Read the model definition and answer for the solid it produces. Units are mm, in the model's axes. A direction names the side the tool comes from. Give positions to 0.01 mm unless a question says otherwise; leave off trailing zeros. Order: outer loops, then holes, each group sorted by start corner. A loop starts at its lowest first (then second) coordinate and runs counter-clockwise, first axis right, second up. Notation, with made-up numbers: (70.25, -19) -> (109.25, -19) arc R23 ccw to (109.25, 3) -> close; hole circle Ø3 at (-25, 69). An arc over 180 degrees is marked (long way). Use one line per item in the form item = value.
```python
from build123d import *

# Parameters (mm, degrees)
SKETCH_1_W               = 44
SKETCH_1_H               = 6.22
EXTRUDE_1_DEPTH          = 0.25
SKETCH_2_W               = 0.25
SKETCH_2_H               = 6.22
EXTRUDE_2_DEPTH          = 1.75
SKETCH_4_W               = 34
SKETCH_4_H               = 0.25
SKETCH_4_W_2             = 9.35
EXTRUDE_3_DEPTH          = 2.25
SKETCH_5_W               = 22.25
SKETCH_5_H               = 2.25
SKETCH_5_W_2             = 9
SKETCH_5_H_2             = 7.53
EXTRUDE_4_DEPTH          = 0.25
SKETCH_6_W               = 21
SKETCH_6_H               = 5.6
EXTRUDE_5_DEPTH          = 0.25
SKETCH_7_W               = 18
SKETCH_7_H               = 2.3
CUT_EXTRUDE_1_DEPTH      = 45.877509958
SKETCH_8_W               = 21
SKETCH_8_H               = 0.25
EXTRUDE_6_DEPTH          = 1.63
SKETCH_9_W               = 28
SKETCH_9_H               = 0.25
EXTRUDE_7_DEPTH          = 2.3
EXTRUDE_8_DEPTH          = 2.3
EXTRUDE_9_DEPTH          = 1.95
SKETCH_12_W              = 2.3
SKETCH_12_H              = 2.401936356
CUT_EXTRUDE_2_DEPTH      = 51.369645687
CUT_EXTRUDE_3_DEPTH      = 49.492266831
CUT_EXTRUDE_3_DEPTH_BACK = 49.492266831
SKETCH_13_W              = 0.7
SKETCH_13_H              = 8.10994941
CUT_EXTRUDE_4_DEPTH      = 0.7
SKETCH_15_W              = 22.25
SKETCH_15_H              = 0.25
EXTRUDE_10_DEPTH         = 2
EXTRUDE_11_DEPTH         = 0.25
CUT_EXTRUDE_5_REACH      = 48.336
SKETCH_17_W              = 4.75
SKETCH_17_H              = 8
SKETCH_18_W              = 3.75
SKETCH_18_H              = 0.25
EXTRUDE_12_DEPTH         = 2.2
EXTRUDE_13_DEPTH         = 0.25


with BuildPart() as part:
    # 草图1 → 凸台-拉伸1 (new body)
    with BuildSketch(Plane(origin=(0, 0, 0), x_dir=(0, 0, -1), z_dir=(1, 0, 0))):
        with Locations((22, 3.11)):
            Rectangle(SKETCH_1_W, SKETCH_1_H)
    extrude(amount=EXTRUDE_1_DEPTH)

    # 草图2 → 凸台-拉伸2 (add)
    with BuildSketch(Plane(origin=(0.25, 0, 0), x_dir=(0, 0, -1), z_dir=(1, 0, 0))):
        with Locations((43.875, 3.11)):
            Rectangle(SKETCH_2_W, SKETCH_2_H)
    extrude(amount=EXTRUDE_2_DEPTH)

    # 草图4 → 凸台-拉伸3 (add)
    with BuildSketch(Plane.ZY):
        with Locations((-27, 0.125)):
            Rectangle(SKETCH_4_W, SKETCH_4_H)
        with Locations((-28.625, 6.095)):
            Rectangle(SKETCH_4_W_2, SKETCH_4_H)
    extrude(amount=EXTRUDE_3_DEPTH)

    # 草图5 → 凸台-拉伸4 (add)
    with BuildSketch(Plane(origin=(0.25, 0, 0), x_dir=(0, 0, -1), z_dir=(1, 0, 0))):
        with Locations((11.125, 7.345)):
            Rectangle(SKETCH_5_W, SKETCH_5_H)
        with Locations((4.5, -3.765)):
            Rectangle(SKETCH_5_W_2, SKETCH_5_H_2)
    extrude(amount=-EXTRUDE_4_DEPTH)

    # 草图6 → 凸台-拉伸5 (add)
    with BuildSketch(Plane(origin=(0.25, 0, 0), x_dir=(0, 0, -1), z_dir=(1, 0, 0))):
        with Locations((-10.5, -4.73)):
            Rectangle(SKETCH_6_W, SKETCH_6_H)
    extrude(amount=-EXTRUDE_5_DEPTH)

    # 草图7 → 切除-拉伸1 (cut, through all)
    with BuildSketch(Plane(origin=(0.25, 0, 0), x_dir=(0, 0, -1), z_dir=(1, 0, 0))):
        with Locations((-12, -6.38)):
            Rectangle(SKETCH_7_W, SKETCH_7_H)
    extrude(amount=-CUT_EXTRUDE_1_DEPTH, mode=Mode.SUBTRACT)

    # 草图8 → 凸台-拉伸6 (add)
    with BuildSketch(Plane(origin=(0.25, 0, 0), x_dir=(0, 0, -1), z_dir=(1, 0, 0))):
        with Locations((-10.5, -2.055)):
            Rectangle(SKETCH_8_W, SKETCH_8_H)
    extrude(amount=EXTRUDE_6_DEPTH)

    # 草图9 → 凸台-拉伸7 (add)
    with BuildSketch(Plane.ZY):
        with Locations((5, -7.405)):
            Rectangle(SKETCH_9_W, SKETCH_9_H)
    extrude(amount=EXTRUDE_7_DEPTH)

    # 草图10 → 凸台-拉伸8 (add)
    with BuildSketch(Plane.ZY.offset(2.3)):
        Polygon((19, -7.28), (24.5, -11.465833127), (24.5, -11.78), (18.91568756, -7.53), (19, -7.53), align=None)
    extrude(amount=-EXTRUDE_8_DEPTH)

    # 草图11 → 凸台-拉伸9 (add)
    with BuildSketch(Plane.ZY.offset(2.3)):
        Polygon((24.5, -11.465833127), (20.919100499, -8.740551717), (20.767695976, -8.939490578), (24.5, -11.78), (30.85, -11.78), (30.85, -11.465833127), align=None)
    extrude(amount=EXTRUDE_9_DEPTH)

    # 草图12 → 切除-拉伸2 (cut, through all)
    with BuildSketch(Plane(origin=(0, 4.546663396, 3.460286229), x_dir=(1, 0, 0), z_dir=(0, 0.795755444677028, 0.6056180910993872))):
        with Locations((-1.15, -25.42922133)):
            Rectangle(SKETCH_12_W, SKETCH_12_H)
    extrude(amount=-CUT_EXTRUDE_2_DEPTH, mode=Mode.SUBTRACT)

    # 草图13 → 切除-拉伸3 (cut, two sides: drawn at the far end of the back side and taken through both)
    with BuildSketch(Plane(origin=(0, -11.465833127, 0), x_dir=(1, 0, 0), z_dir=(0, 1, 0)).offset(-CUT_EXTRUDE_3_DEPTH_BACK)):
        with Locations((-2.65, -26.795025295)):
            Rectangle(SKETCH_13_W, SKETCH_13_H)
    extrude(amount=CUT_EXTRUDE_3_DEPTH + CUT_EXTRUDE_3_DEPTH_BACK, mode=Mode.SUBTRACT)

    # 草图14 → 切除-拉伸4 (cut)
    with BuildSketch(Plane(origin=(-2.3, 0, 0), x_dir=(0, 0, -1), z_dir=(1, 0, 0))):
        Polygon((-22.74005059, -10.126405028), (-22.74005059, -10.440571902), (-22.588646067, -10.325343889), align=None)
    extrude(amount=-CUT_EXTRUDE_4_DEPTH, mode=Mode.SUBTRACT)

    # 草图15 → 凸台-拉伸10 (add)
    with BuildSketch(Plane.ZY):
        with Locations((-11.125, 8.345)):
            Rectangle(SKETCH_15_W, SKETCH_15_H)
    extrude(amount=EXTRUDE_10_DEPTH)

    # 草图16 → 凸台-拉伸11 (add)
    with BuildSketch(Plane.XY):
        Polygon((0, 2.82), (0, 8.22), (-2, 8.22), (-2, 8.47), (0, 8.47), (0, 10.82), (-8.5, 10.82), (-5, 2.82), align=None)
    extrude(amount=-EXTRUDE_11_DEPTH)

    # 草图17 → 切除-拉伸5 (cut, up to next)
    with BuildSketch(Plane.XY, mode=Mode.PRIVATE) as cut_extrude_5_sk1:
        with Locations((-6.125, 6.82)):
            Rectangle(SKETCH_17_W, SKETCH_17_H)
    cut_extrude_5_tool1 = extrude(cut_extrude_5_sk1.sketch, amount=-CUT_EXTRUDE_5_REACH, mode=Mode.PRIVATE) & part.part
    add(cut_extrude_5_tool1.solids().sort_by_distance((-6.125, 6.82, 0))[0], mode=Mode.SUBTRACT)

    # 草图18 → 凸台-拉伸12 (add)
    with BuildSketch(Plane.XY):
        with Locations((-1.875, 2.945)):
            Rectangle(SKETCH_18_W, SKETCH_18_H)
    extrude(amount=EXTRUDE_12_DEPTH)

    # 草图19 → 凸台-拉伸13 (add)
    with BuildSketch(Plane.ZY.offset(3.75)):
        Polygon((0, 10.82), (5, 10.82), (4, 3.57), (0, 3.57), align=None)
    extrude(amount=-EXTRUDE_13_DEPTH)


solid = part.part
```
Item 1: Given pin 1 Ø1.6 at (y, z) = (8, 3.5) entering from -X; pin 2 Ø2 at (x, y) = (-2, -8) entering from +Z; pin 3 Ø1.8 at (x, z) = (-0.5, -9) entering from +Y; pin 4 Ø1.8 at (y, z) = (-8.5, 5) entering from -X, each flat-ended and moving along its own axis, determine where each tip first touches the part or whether it passes through.
Checks:
pin_1 = -3.75
pin_2 = 21.26
pin_3 = 8.47
pin_4 = through
Item 2: The part is cut by section D-D on y = -1. Give the vertices of the cut face in (x, z), and give its area (3 significant figures).
Checks:
outline = (0, -9) -> (0.25, -9) -> (0.25, 0) -> (0, 0) -> close
area = 2.25 mm²
Item 3: Straight lines are drawn through the part: L1, parallel to Y at x = -1, z = -33; L2, parallel to X at y = 2, z = -0.5; L3, parallel to Z at x = -0.75, y = 4.25. For each, find the intervals that lie inside material, in ascending order. Write a range as from..to.
Checks:
L1 = 0..0.25, 5.97..6.22
L2 = 0..0.25
L3 = -0.25..0
Item 4: The part is cut by section B-B on z = -3. Give the vertices of the cut face in (x, y), and give its area (4 significant figures).
Checks:
outline = (-2.3, -7.53) -> (0.25, -7.53) -> (0.25, 8.47) -> (-2, 8.47) -> (-2, 8.22) -> (0, 8.22) -> (0, -7.28) -> (-2.3, -7.28) -> close
area = 5.075 mm²
Item 5: Which of the six approach directions +Z, -Z, +X, -X, +Y, -Y give full straight-line access (tool end or side, diameter ignored) to faces 1 (the flat face through (-1, 6.22, -30)), 2 (the flat face through (1, -2.18, 11)), 3 (the flat face through (-1, 8.22, -11)), 4 (the flat face through (-4, -11.466, 28))?
Checks:
face_1 = -Z, +X, -X, +Y
face_2 = +Z, -Z, +X, -Y
face_3 = -Z, -X
face_4 = +Z, +X, -X, +Y
Item 6: Determine the mould class of faces 5 (the flat face through (-1, 0, -27)), 6 (the flat face through (0.25, 2, -11)), 7 (the flat face through (-1, 5.97, -29)) for opening direction Y: +Y half, -Y half, draft (parallel to the pull), parting line (faces both ways), or undercut.
Checks:
face_5 = -Y half
face_6 = draft
face_7 = undercut
Item 7: The part is cut by section C-C on y = 7.25. Give the vertices of the cut face in (x, z), and give its area (3 significant figures).
Checks:
outline = (-3.75, -0.25) -> (0, -0.25) -> (0, -22.25) -> (0.25, -22.25) -> (0.25, 0) -> (-3.5, 0) -> (-3.5, 4.51) -> (-3.75, 4.51) -> close
area = 7.63 mm²
Item 8: The part is cut by section A-A on z = 15. Give the vertices of the cut face in (x, y), and give its area (3 significant figures).
Checks:
outline = (-2.3, -7.53) -> (0, -7.53) -> (0, -7.28) -> (-2.3, -7.28) -> close; (0, -5.23) -> (0.25, -5.23) -> (0.25, -2.18) -> (1.88, -2.18) -> (1.88, -1.93) -> (0, -1.93) -> close
area = 1.81 mm²
